from build123d import *

# Parameters (mm, degrees)
SKETCH1_R           = 4
BOSS_EXTRUDE1_DEPTH = 10
SKETCH2_R           = 4
SKETCH2_R_2         = 2.5
BOSS_EXTRUDE2_DEPTH = 2


with BuildPart() as part:
    # Sketch1 → Boss-Extrude1 (new body)
    with BuildSketch(Plane(origin=(0, 0, 0), x_dir=(1, 0, 0), z_dir=(0, 1, 0))):
        with Locations(Location((0, 0, 0), (0, 0, 270))):
            Circle(SKETCH1_R)
        with BuildLine():
            Line((-1.341640786, 1.55), (1.341640786, 1.55))
            ThreePointArc((1.341640786, 1.55), (0, -2.05), (-1.341640786, 1.55))
        make_face(mode=Mode.SUBTRACT)
    extrude(amount=BOSS_EXTRUDE1_DEPTH)

    # Sketch2 → Boss-Extrude2 (add)
    with BuildSketch(Plane(origin=(0, 10, 0), x_dir=(1, 0, 0), z_dir=(0, 1, 0))):
        with Locations(Location((0, 0, 0), (0, 0, 270))):
            Circle(SKETCH2_R)
        with Locations(Location((0, 0, 0), (0, 0, 270))):
            Circle(SKETCH2_R_2, mode=Mode.SUBTRACT)
    extrude(amount=BOSS_EXTRUDE2_DEPTH)


solid = part.part
Here's how the part is built. I have some questions about the finished solid (model axes, mm). A direction names the side the tool comes from. Give positions to 0.01 mm unless a question says otherwise; leave off trailing zeros. Order: outer loops, then holes, each group sorted by start corner. A loop starts at its lowest first (then second) coordinate and runs counter-clockwise, first axis right, second up. Notation, with made-up numbers: (-11.5, -10.5) -> (30.5, -10.5) arc R5 cw to (30.5, -6.5) -> close; hole circle Ø7 at (24, 47). An arc over 180 degrees is marked (long way). One line per item, written item: value. Start each with the question number.
1. I need wall thicknesses on probe 1 along X at (y, z) = (11.35, 0); probe 2 along X at (y, z) = (6.25, 0); probe 3 along Y at (x, z) = (-0.5, -1.75). Which ranges of each line are inside material? Lowest first, please. Write a range as from..to.
2. Imagine slicing it at C-C, the plane y = 9.5. List the corners of the cut face in (x, z) for me.
3. Imagine slicing it at D-D, the plane z = -1.75. List the corners of the cut face in (x, y) for me.
4. We'd pull the mould along Z, two halves only. Please class faces 3 (the face through (0, 5, -1.55)), 4 (the face through (2, 12, 2)), 5 (the face through (-3.905, 5.916, -0.867)): released by +Z, released by -Z, zero draft, split by the parting line, or undercut.
5. For faces 1 (the face through (0, 10, -2)), 2 (the face through (0, 0, -2)), which set-ups out of +Z, -Z, +X, -X, +Y, -Y let a thin tool reach every point of the face, with its end or its side?
6. Imagine slicing it at B-B, the plane z = 0.75. List the corners of the cut face in (x, y) for me.
7. Will these pins go through, and if not, where does the flat tip stop? pin 1 Ø3 at (y, z) = (3, -0.5) entering from -X; pin 2 Ø1 at (x, y) = (2.5, 6) entering from +Z.
8. Imagine slicing it at A-A, the plane x = 0. List the corners of the cut face in (y, z) for me.
Values follow:
1. probe 1: x = -4..-2.5, 2.5..4
1. probe 2: x = -4..-2.05, 2.05..4
1. probe 3: y = 0..10
2. outline: circle Ø8 at (0, 0); hole (-1.34, -1.55) -> (1.34, -1.55) arc R2.05 ccw (long way) to start
3. outline: (-3.6, 0) -> (3.6, 0) -> (3.6, 12) -> (1.79, 12) -> (1.79, 10) -> (-1.79, 10) -> (-1.79, 12) -> (-3.6, 12) -> close
4. face 3: undercut
4. face 4: zero draft
4. face 5: split by the parting line
5. face 1: +Y
5. face 2: +Z, -Z, +X, -X, -Y
6. outline: (-3.93, 0) -> (-1.91, 0) -> (-1.91, 10) -> (-2.38, 10) -> (-2.38, 12) -> (-3.93, 12) -> close; (1.91, 0) -> (3.93, 0) -> (3.93, 12) -> (2.38, 12) -> (2.38, 10) -> (1.91, 10) -> close
7. pin 1: stops at x = -4
7. pin 2: stops at z = 3.46
8. outline: (0, -4) -> (12, -4) -> (12, -2.5) -> (10, -2.5) -> (10, -1.55) -> (0, -1.55) -> close; (0, 2.05) -> (10, 2.05) -> (10, 2.5) -> (12, 2.5) -> (12, 4) -> (0, 4) -> close
